from build123d import *

# Parameters (mm, degrees)
F1_DEPTH = 101.6
F3_D     = 6.35


with BuildPart() as f1:
    # F0 (on Top) → F1 (new body)
    with BuildSketch(Plane.XY):
        Polygon((0, 0), (-19.05, 0), (-19.05, -3.175), (-3.175, -3.175), (-3.175, -50.8), (0, -50.8), align=None)
    extrude(amount=F1_DEPTH)

    # F3 (through all)
    with Locations(Plane(origin=(0, 0, 0), x_dir=(1, 0, 0), z_dir=(0, 1, 0))):
        with Locations((-10.5969142169, -29.7635085881)):
            Hole(F3_D / 2)


solid = f1.part
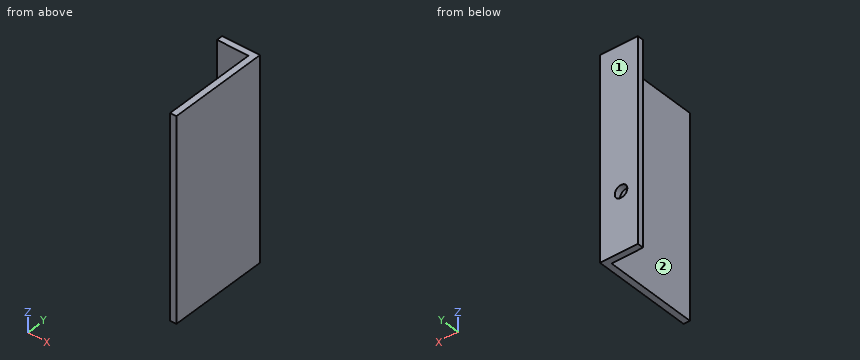
Input: part model. Units: mm. Frame: model coordinates. Face numbers are marked on the shaded views. A direction names the side the tool comes from. Round coordinates to 2 decimals unless told otherwise and drop trailing zeros. Loops run counter-clockwise (first coordinate to the right, second up) from the corner with the lowest first, then second, coordinate; pieces in that order, holes last. Notation, with made-up numbers: M 61.5,4.25 L 83.5,4.25 A12 cw 83.5,19.25 Z; hole C -12.75,24 d10. An arc over 180 degrees is marked long. Answer as CSV lines item,"result". Start each with the question number.
(1) Section A-A, the plane x = -12. Output: boundary loops of the cut face in (y, z) (3 decimals), plus the area to 3 significant figures.
(2) Line query: line 1 (X direction, y = -7, z = 88) (3 decimals). Output: solid intervals per line, ascending. Write a range as [from, to].
(3) First-contact query: pin 1 (24 mm diameter, centred on y = -20, z = 38, fed in from -X) (3 decimals); pin 2 (12 mm diameter, centred on y = -25.5, z = 40, fed in from +X); pin 3 (8.5 mm diameter, centred on x = -10.6, z = 29.76, fed in from -Y) (3 decimals). Flat tips, straight axial feed; report the tip coordinate or a pass-through.
(4) Section B-B, the plane z = 72.5. Output: boundary loops of the cut face in (x, y) (3 decimals), plus the area to 3 significant figures.
(5) Reachability of the marked faces 1 and 2 from +Z, -Z, +X, -X, +Y, -Y: full face, straight path, thin tool, end or side. Return the list, or none.
(6) Section C-C, the plane y = -9. Output: boundary loops of the cut face in (x, z) (3 decimals).
Values found:
1,outline,"M -3.175,0 L 0,0 L 0,26.915 L -3.175,26.915 Z; M -3.175,32.612 L 0,32.612 L 0,101.6 L -3.175,101.6 Z"
1,area,"304 mm²"
2,line 1,"x = [-3.175, 0]"
3,pin 1,"stops at x = -3.175"
3,pin 2,"stops at x = 0"
3,pin 3,"stops at y = -3.175"
4,outline,"M -19.05,-3.175 L -3.175,-3.175 L -3.175,-50.8 L 0,-50.8 L 0,0 L -19.05,0 Z"
4,area,"212 mm²"
5,face 1,"+Z, -Z, +X, -X, +Y"
5,face 2,"+Z, -Z, -X, -Y"
6,outline,"M -3.175,0 L 0,0 L 0,101.6 L -3.175,101.6 Z"
